```python
from build123d import *

# Parameters (mm, degrees)
SKETCH1_W            = 110
SKETCH1_H            = 45
BOSS_EXTRUDE1_DEPTH  = 46.5
SKETCH2_W            = 100
SKETCH2_H            = 42
CUT_EXTRUDE1_DEPTH   = 41.5
SKETCH24_W           = 3
SKETCH24_H           = 1
CUT_EXTRUDE10_DEPTH  = 41.5
SKETCH26_W           = 10
SKETCH26_H           = 10
SKETCH26_H_2         = 13.5
BOSS_EXTRUDE2_DEPTH  = 41.5
M3_CLEARANCE_HOLE5_D = 3.4
SKETCH29_W           = 10
SKETCH29_H           = 27.5
SKETCH29_W_2         = 13.5
CUT_EXTRUDE11_DEPTH  = 9
SKETCH30_W           = 10
SKETCH30_H           = 27.5
SKETCH30_W_2         = 13.5
CUT_EXTRUDE12_DEPTH  = 9
SKETCH32_W           = 3
SKETCH32_H           = 1
CUT_EXTRUDE14_DEPTH  = 41.5
SKETCH33_W           = 1
SKETCH33_H           = 3
CUT_EXTRUDE15_DEPTH  = 41.5
SKETCH34_W           = 98
SKETCH34_H           = 5
CUT_EXTRUDE16_DEPTH  = 1


with BuildPart() as part:
    # Sketch1 → Boss-Extrude1 (new body)
    with BuildSketch(Plane(origin=(0, 0, 0), x_dir=(1, 0, 0), z_dir=(0, 1, 0))):
        with Locations((55, 22.5)):
            Rectangle(SKETCH1_W, SKETCH1_H)
    extrude(amount=BOSS_EXTRUDE1_DEPTH)

    # Sketch2 → Cut-Extrude1 (cut)
    with BuildSketch(Plane(origin=(0, 46.5, 0), x_dir=(1, 0, 0), z_dir=(0, 1, 0))):
        with Locations((55, 21)):
            Rectangle(SKETCH2_W, SKETCH2_H)
    extrude(amount=-CUT_EXTRUDE1_DEPTH, mode=Mode.SUBTRACT)

    # Sketch24 → Cut-Extrude10 (cut)
    with BuildSketch(Plane(origin=(0, 46.5, 0), x_dir=(1, 0, 0), z_dir=(0, 1, 0))):
        with Locations((55, 42.5)):
            Rectangle(SKETCH24_W, SKETCH24_H)
    extrude(amount=-CUT_EXTRUDE10_DEPTH, mode=Mode.SUBTRACT)

    # Sketch26 → Boss-Extrude2 (add)
    with BuildSketch(Plane(origin=(0, 5, 0), x_dir=(1, 0, 0), z_dir=(0, 1, 0))):
        with Locations((10, 37)):
            Rectangle(SKETCH26_W, SKETCH26_H)
        with Locations((10, 6.75)):
            Rectangle(SKETCH26_W, SKETCH26_H_2)
        with Locations((100, 37)):
            Rectangle(SKETCH26_W, SKETCH26_H)
        with Locations((100, 6.75)):
            Rectangle(SKETCH26_W, SKETCH26_H_2)
    extrude(amount=BOSS_EXTRUDE2_DEPTH)

    # M3 Clearance Hole5 (through all)
    with Locations(Plane(origin=(0, 46.5, 0), x_dir=(1, 0, 0), z_dir=(0, 1, 0))):
        with Locations((10.295, 36.91), (99.705, 36.91), (99.705, 8.97), (10.295, 8.97)):
            Hole(M3_CLEARANCE_HOLE5_D / 2)

    # Sketch29 → Cut-Extrude11 (cut)
    with BuildSketch(Plane(origin=(15, 0, 0), x_dir=(0, 0, -1), z_dir=(1, 0, 0))):
        with Locations((37, 25.75)):
            Rectangle(SKETCH29_W, SKETCH29_H)
        with Locations((6.75, 25.75)):
            Rectangle(SKETCH29_W_2, SKETCH29_H)
    extrude(amount=-CUT_EXTRUDE11_DEPTH, mode=Mode.SUBTRACT)

    # Sketch30 → Cut-Extrude12 (cut)
    with BuildSketch(Plane.ZY.offset(-95)):
        with Locations((-37, 25.75)):
            Rectangle(SKETCH30_W, SKETCH30_H)
        with Locations((-6.75, 25.75)):
            Rectangle(SKETCH30_W_2, SKETCH30_H)
    extrude(amount=-CUT_EXTRUDE12_DEPTH, mode=Mode.SUBTRACT)

    # Sketch32 → Cut-Extrude14 (cut)
    with BuildSketch(Plane(origin=(0, 46.5, 0), x_dir=(1, 0, 0), z_dir=(0, 1, 0))):
        with Locations((17.198, 42.5)):
            Rectangle(SKETCH32_W, SKETCH32_H)
        with Locations((92.802, 42.5)):
            Rectangle(SKETCH32_W, SKETCH32_H)
    extrude(amount=-CUT_EXTRUDE14_DEPTH, mode=Mode.SUBTRACT)

    # Sketch33 → Cut-Extrude15 (cut)
    with BuildSketch(Plane(origin=(0, 46.5, 0), x_dir=(1, 0, 0), z_dir=(0, 1, 0))):
        with Locations((4.5, 15.55)):
            Rectangle(SKETCH33_W, SKETCH33_H)
        with Locations((105.5, 15.55)):
            Rectangle(SKETCH33_W, SKETCH33_H)
    extrude(amount=-CUT_EXTRUDE15_DEPTH, mode=Mode.SUBTRACT)

    # Sketch34 → Cut-Extrude16 (cut)
    with BuildSketch(Plane.XY.offset(-42)):
        with Locations((55, 14.5)):
            Rectangle(SKETCH34_W, SKETCH34_H)
    extrude(amount=-CUT_EXTRUDE16_DEPTH, mode=Mode.SUBTRACT)


solid = part.part
```
Part model, mm, in its own coordinate system. A direction names the side the tool comes from. Round coordinates to 2 decimals unless told otherwise and drop trailing zeros. Order: outer loops, then holes, each group sorted by start corner. A loop starts at its lowest first (then second) coordinate and runs counter-clockwise, first axis right, second up. Notation, with made-up numbers: M -3,-6 L 5,-6 A30 cw 5,20 Z; hole C 57.25,8 d1. An arc over 180 degrees is marked long. Put each result on its own line as item: value. Start each with the question number.
1. Drill centre lines: probe 1 along X at (y, z) = (42.25, -8.97) (3 decimals); probe 2 along X at (y, z) = (6, -6.5); probe 3 along X at (y, z) = (3, -8.97) (3 decimals). Where is each one in solid material? Low to high. Write a range as [from, to].
2. Slice it at C-C on z = -3. List the corners of the cut face in (x, y), then the cut area to 3 significant figures.
3. Tool access for faces 5 (the face through (11, 12, -7)), 6 (the face through (74, 9, -42)), 7 (the face through (5.5, 20.8, -13.5)): list every direction of +Z, -Z, +X, -X, +Y, -Y with a clear straight run to the whole face (end or side of a thin tool).
4. Slice it at B-B on x = 71.5. List the corners of the cut face in (y, z).
5. Slice it at A-A on z = -36.91. State how many separate pieces and enclosed holes the cut face has, then the cut area to 3 significant figures.
6. Slice it at D-D on x = 55. List the corners of the cut face in (y, z).
7. Two-plate mould, pull along Y, no slides. Class faces 1 (the face through (99, 29, -42)), 2 (the face through (6, 26, -7)), 3 (the face through (4, 26, -16)), 4 (the face through (55, 46.5, -44)): +Y half, -Y half, draft (parallel to the pull), parting line (faces both ways), or undercut.
8. Drop flat-ended pins along their axis: pin 1 (3.5 mm diameter, centred on x = 43, y = 7, fed in from +Z); pin 2 (3 mm diameter, centred on x = 89, z = -27.5, fed in from -Y); pin 3 (2 mm diameter, centred on x = 20.5, z = -18.5, fed in from +Y). Give the stop position or say it passes through.
Findings:
1. probe 1: [0, 8.595], [11.995, 15], [95, 98.005], [101.405, 110]
1. probe 2: [0, 15], [95, 110]
1. probe 3: [0, 8.595], [11.995, 98.005], [101.405, 110]
2. outline: M 0,0 L 110,0 L 110,46.5 L 95,46.5 L 95,39.5 L 104,39.5 L 104,12 L 95,12 L 95,5 L 15,5 L 15,12 L 6,12 L 6,39.5 L 15,39.5 L 15,46.5 L 0,46.5 Z
2. area: 1,300 mm2
3. face 5: +Z
3. face 6: +Z, +Y
3. face 7: +Y
4. outline: M 0,-45 L 46.5,-45 L 46.5,-42 L 17,-42 L 17,-43 L 12,-43 L 12,-42 L 5,-42 L 5,0 L 0,0 Z
5. separate pieces: 5
5. enclosed holes: 0
5. area: 1,170 mm2
6. outline: M 0,-45 L 46.5,-45 L 46.5,-43 L 5,-43 L 5,0 L 0,0 Z
7. face 1: undercut
7. face 2: undercut
7. face 3: draft
7. face 4: +Y half
8. pin 1: z = -42
8. pin 2: y = 0
8. pin 3: y = 5
